```python
from build123d import *

# Parameters (mm, degrees)
SKETCH1_W           = 74
SKETCH1_H           = 24
SKETCH1_W_2         = 68
SKETCH1_H_2         = 18
BOSS_EXTRUDE1_DEPTH = 20
SKETCH1_3_W         = 74
SKETCH1_3_H         = 24
SKETCH1_3_W_2       = 68
SKETCH1_3_H_2       = 18
BOSS_EXTRUDE2_DEPTH = 3
CUT_EXTRUDE1_REACH  = 61.463
SKETCH4_W           = 18
SKETCH4_H           = 10
SKETCH5_W           = 7.9
SKETCH5_H           = 23
BOSS_EXTRUDE3_DEPTH = 9.2


with BuildPart() as part:
    # Sketch1 → Boss-Extrude1 (new body)
    with BuildSketch(Plane(origin=(0, 0, 0), x_dir=(1, 0, 0), z_dir=(0, 1, 0))):
        with Locations((14.912280702, -12.336842105)):
            Rectangle(SKETCH1_W, SKETCH1_H)
        with Locations((14.912280702, -12.336842105)):
            Rectangle(SKETCH1_W_2, SKETCH1_H_2, mode=Mode.SUBTRACT)
    extrude(amount=BOSS_EXTRUDE1_DEPTH)

    # Sketch1_3 → Boss-Extrude2 (add)
    # profile 1 of 2: a face of its own
    with BuildSketch(Plane(origin=(0, 0, 0), x_dir=(1, 0, 0), z_dir=(0, 1, 0))):
        with Locations((14.912280702, -12.336842105)):
            Rectangle(SKETCH1_3_W, SKETCH1_3_H)
        with Locations((14.912280702, -12.336842105)):
            Rectangle(SKETCH1_3_W_2, SKETCH1_3_H_2, mode=Mode.SUBTRACT)
    # profile 2 of 2: a face of its own
    with BuildSketch(Plane(origin=(0, 0, 0), x_dir=(1, 0, 0), z_dir=(0, 1, 0))):
        with Locations((14.912280702, -12.336842105)):
            Rectangle(SKETCH1_3_W_2, SKETCH1_3_H_2)
    extrude(amount=-BOSS_EXTRUDE2_DEPTH)

    # Sketch4 → Cut-Extrude1 (cut, up to next)
    with BuildSketch(Plane(origin=(0, 0, 21.336842105), x_dir=(-1, 0, 0), z_dir=(0, 0, -1)), mode=Mode.PRIVATE) as cut_extrude1_sk1:
        with Locations((-14.912280702, 15)):
            Rectangle(SKETCH4_W, SKETCH4_H)
    cut_extrude1_tool1 = extrude(cut_extrude1_sk1.sketch, amount=-CUT_EXTRUDE1_REACH, mode=Mode.PRIVATE) & part.part
    add(cut_extrude1_tool1.solids().sort_by_distance((14.912281, 15, 21.336842))[0], mode=Mode.SUBTRACT)

    # Sketch5 → Boss-Extrude3 (add)
    with BuildSketch(Plane(origin=(0, 0, 0.336842105), x_dir=(-1, 0, 0), z_dir=(0, 0, -1))):
        with Locations((-14.912280702, 8.5)):
            Rectangle(SKETCH5_W, SKETCH5_H)
    extrude(amount=BOSS_EXTRUDE3_DEPTH)


solid = part.part
```
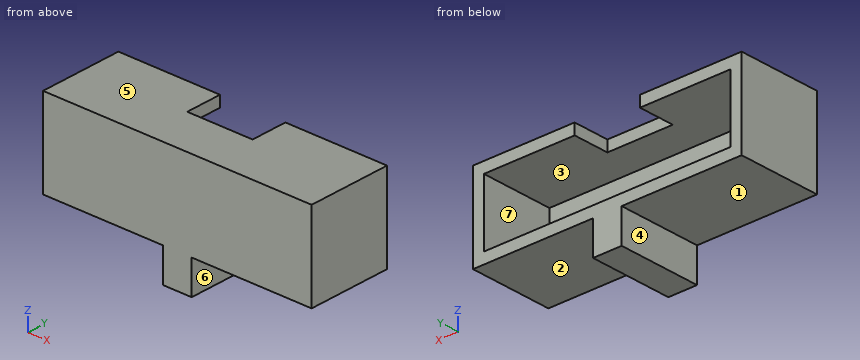
Design review of the part built by this model. Coordinates are the model's own, in mm. Face numbers are marked on the shaded views. A direction names the side the tool comes from. Give positions to 0.01 mm unless a question says otherwise; leave off trailing zeros. Order: outer loops, then holes, each group sorted by start corner. A loop starts at its lowest first (then second) coordinate and runs counter-clockwise, first axis right, second up. Notation, with made-up numbers: (43, 41) -> (47, 41) arc R14 cw to (47, 59) -> close; hole circle Ø2 at (23, 26). An arc over 180 degrees is marked (long way). Write item = value, one per line. Start each with the question number.
(1) For pin 1 (11.5 mm diameter, centred on x = 43, y = 10, fed in from -Z); pin 2 (3.5 mm diameter, centred on x = 11.5, z = 23, fed in from +Y); pin 3 (10 mm diameter, centred on y = 4.5, z = -6.5, fed in from +X), all flat-tipped, find the tip position at first contact; note any pin that passes through.
(2) We need section D-D on z = 14. Write out the cut boundary in (x, y), plus the area to 3 significant figures.
(3) Mouldability with a two-part tool opening along X and no side actions: class the marked faces 4, 5, 6 and 7 as +X half, -X half, draft (parallel to the pull), parting line (faces both ways), or undercut.
(4) We need section B-B on y = 18. Write out the cut boundary in (x, z).
(5) To check wall thickness, follow line 1 along X through (y, z) = (16.5, 19); line 2 along Z through (x, y) = (-18, 11.5); line 3 along X through (y, z) = (11.5, 22). State the ranges of each line that lie inside material, in increasing order.
(6) For the marked faces 1, 2 and 3, list the 3-axis set-ups (+Z, -Z, +X, -X, +Y, -Y) from which the entire face can be reached by the end or side of a thin tool; tool diameter is ignored.
(7) We need section A-A on y = 6. Write out the cut boundary in (x, z), plus the area to 3 significant figures.
(8) We need section C-C on x = -8. Write out the cut boundary in (y, z).
Numbers:
q1.pin_1 = 0.34
q1.pin_2 = 10
q1.pin_3 = 18.86
q2.outline = (-22.09, -3) -> (51.91, -3) -> (51.91, 20) -> (48.91, 20) -> (48.91, 0) -> (-19.09, 0) -> (-19.09, 20) -> (-22.09, 20) -> close
q2.area = 342 mm^2
q3.face_4 = -X half
q3.face_5 = draft
q3.face_6 = +X half
q3.face_7 = undercut
q4.outline = (-22.09, 0.34) -> (10.96, 0.34) -> (10.96, -8.86) -> (18.86, -8.86) -> (18.86, 0.34) -> (51.91, 0.34) -> (51.91, 24.34) -> (23.91, 24.34) -> (23.91, 21.34) -> (48.91, 21.34) -> (48.91, 3.34) -> (-19.09, 3.34) -> (-19.09, 21.34) -> (5.91, 21.34) -> (5.91, 24.34) -> (-22.09, 24.34) -> close
q5.line_1 = -22.09 to -19.09, 48.91 to 51.91
q5.line_2 = 0.34 to 3.34, 21.34 to 24.34
q5.line_3 = -22.09 to 5.91, 23.91 to 51.91
q6.face_1 = -Z, -X, +Y, -Y
q6.face_2 = -Z, +X, +Y, -Y
q6.face_3 = +Y
q7.outline = (-22.09, 0.34) -> (10.96, 0.34) -> (10.96, -8.86) -> (18.86, -8.86) -> (18.86, 0.34) -> (51.91, 0.34) -> (51.91, 24.34) -> (-22.09, 24.34) -> close; hole (-19.09, 3.34) -> (48.91, 3.34) -> (48.91, 21.34) -> (-19.09, 21.34) -> close
q7.area = 625 mm^2
q8.outline = (-3, 0.34) -> (20, 0.34) -> (20, 3.34) -> (0, 3.34) -> (0, 21.34) -> (20, 21.34) -> (20, 24.34) -> (-3, 24.34) -> close
